Build history of the part. All positions in model axes, mm. A direction names the side the tool comes from. Give positions to 0.01 mm unless a question says otherwise; leave off trailing zeros. Loops run counter-clockwise (first coordinate to the right, second up) from the corner with the lowest first, then second, coordinate; pieces in that order, holes last.
1) Two-plate mould, pull along Z, no slides. Class faces 3 (the flat face through (-5.836, -5, -16)), 4 (the cylindrical face through (-6.44, 63.89, -17.02)), 5 (the flat face through (-29, -6, 0)), 6 (the cylindrical face through (-6.428, -82.873, -27.291)): +Z half, -Z half, draft (parallel to the pull), parting line (faces both ways), or undercut.
2) 3-axis set-ups, long thin cutter, end or side, ignore diameter. For faces 1 (the flat face through (-29, -6, -1.2)), 2 (the cylindrical face through (-51.63, 75.05, -16.89)): which of +Z, -Z, +X, -X, +Y, -Y reach the whole face in a straight line?
3) Flat gauge pins, fed straight in: P1, Ø0.6, axis at x = -6.5, y = 48.5, coming from the +Z side; P2, Ø1, axis at x = -29, z = -0.5, coming from the +Y side; P3, Ø6, axis at x = -34.5, y = -4.5, coming from the -Z side. Where does each tip first touch, or does it go through?
4) Band-saw the part on A-A on y = 20. List the corners of the cut face in (x, z), then the cut area to 3 significant figures.
5) Band-saw the part on B-B on x = -33. List the corners of the cut face in (y, z).
6) Wall check: line 1 (X direction, y = -3, z = -16.5); line 2 (Z direction, x = -39, y = -20). Give the ranges that are in metal, low to high.
```python
from build123d import *

# Parameters (mm, degrees)
SKETCH_1_W                         = 44
SKETCH_1_H                         = 100
SM_BASE_FLANGE_1_DEPTH             = 1.2
SM_EDGE_FLANGE_2_STRIP_W           = 6.2732
SM_EDGE_FLANGE_2_STRIP_H           = 1.2
SM_EDGE_FLANGE_2_STRIP_CUT_DEPTH   = 100
SM_EDGE_FLANGE_2_STRIP_2_W         = 6.2732
SM_EDGE_FLANGE_2_STRIP_2_H         = 1.2
SM_EDGE_FLANGE_2_STRIP_CUT_2_DEPTH = 100
SM_EDGE_FLANGE_2_DEPTH             = 100
SM_EDGE_FLANGE_2_BEND_DEPTH        = 100
EXTRUDE_1_DEPTH                    = 1.2
EXTRUDE_START                      = -1.2
EXTRUDE_2_DEPTH                    = 1.2
SKETCH_44_R                        = 3.5
CUT_EXTRUDE_3_DEPTH                = 94.590588423
SKETCH_45_W                        = 1.2
SKETCH_45_H                        = 29.2634
EXTRUDE_3_DEPTH                    = 30
SKETCH_48_R                        = 3.5
CUT_EXTRUDE_4_DEPTH                = 104.065268641
FILLET_1_R                         = 13


# Sheet-metal steps are written as plain solids
with BuildPart() as part:
    # Sketch 1 → 基材-凸緣1 (new body)
    with BuildSketch(Plane.XY):
        with Locations((-29.036181479, -6.57972973)):
            Rectangle(SKETCH_1_W, SKETCH_1_H)
    extrude(amount=-SM_BASE_FLANGE_1_DEPTH)

    # 邊線-凸緣2 strip (across the edge) → 邊線-凸緣2 strip cut (cut)
    with BuildSketch(Plane(origin=(-7.036181479, 43.42027027, -1.2), x_dir=(-1, 0, 0), z_dir=(0, -1, 0))):
        with Locations((-2.4, -0.6)):
            Rectangle(SM_EDGE_FLANGE_2_STRIP_W, SM_EDGE_FLANGE_2_STRIP_H)
    extrude(amount=SM_EDGE_FLANGE_2_STRIP_CUT_DEPTH, mode=Mode.SUBTRACT)

    # 邊線-凸緣2 strip 2 (across the edge) → 邊線-凸緣2 strip cut 2 (cut)
    with BuildSketch(Plane(origin=(-51.036181479, -56.57972973, -1.2), x_dir=(1, 0, 0), z_dir=(0, 1, 0))):
        with Locations((-2.4, -0.6)):
            Rectangle(SM_EDGE_FLANGE_2_STRIP_2_W, SM_EDGE_FLANGE_2_STRIP_2_H)
    extrude(amount=SM_EDGE_FLANGE_2_STRIP_CUT_2_DEPTH, mode=Mode.SUBTRACT)

    # 邊線-凸緣2 section (across the edge) → 邊線-凸緣2 (add)
    with BuildSketch(Plane(origin=(-7.036181479, 43.42027027, -1.2), x_dir=(-1, 0, 0), z_dir=(0, -1, 0))):
        with BuildLine():
            Line((-1.2, 0.7366), (-1.2, 30))
            Line((-1.2, 30), (0, 30))
            Line((0, 30), (0, 0.7366))
            ThreePointArc((0, 0.7366), (0.215745145, 0.215745145), (0.7366, 0))
            Line((0.7366, 0), (0.7366, -1.2))
            ThreePointArc((0.7366, -1.2), (-0.632782992, -0.632782992), (-1.2, 0.7366))
        make_face()
    extrude(amount=SM_EDGE_FLANGE_2_DEPTH)

    # 邊線-凸緣2 section 2 (across the edge) → 邊線-凸緣2 bend (add)
    with BuildSketch(Plane(origin=(-51.036181479, -56.57972973, -1.2), x_dir=(1, 0, 0), z_dir=(0, 1, 0))):
        with BuildLine():
            Line((-1.2, 0.7366), (-1.2, 30))
            Line((-1.2, 30), (0, 30))
            Line((0, 30), (0, 0.7366))
            ThreePointArc((0, 0.7366), (0.215745145, 0.215745145), (0.7366, 0))
            Line((0.7366, 0), (0.7366, -1.2))
            ThreePointArc((0.7366, -1.2), (-0.632782992, -0.632782992), (-1.2, 0.7366))
        make_face()
    extrude(amount=SM_EDGE_FLANGE_2_BEND_DEPTH)

    # 草圖38 → 填料-伸長1 (add)
    with BuildSketch(Plane(origin=(-5.836181479, 0, 0), x_dir=(0, 0, -1), z_dir=(1, 0, 0))):
        with BuildLine():
            Line((1.9366, 43.42027027), (31.2, 43.42027027))
            Line((31.2, 43.42027027), (31.2, 60.42027027))
            ThreePointArc((31.2, 60.42027027), (16.5683, 75.05197027), (1.9366, 60.42027027))
            Line((1.9366, 60.42027027), (1.9366, 43.42027027))
        make_face()
    extrude(amount=-EXTRUDE_1_DEPTH)

    # 草圖41 → 填料-伸長2 (add)
    with BuildSketch(Plane.ZY.offset(52.236181479).offset(EXTRUDE_START)):
        with BuildLine():
            Line((-1.9366, 43.42027027), (-31.2, 43.42027027))
            Line((-31.2, 43.42027027), (-31.2, 60.42027027))
            ThreePointArc((-31.2, 60.42027027), (-16.5683, 75.05197027), (-1.9366, 60.42027027))
            Line((-1.9366, 60.42027027), (-1.9366, 43.42027027))
        make_face()
    extrude(amount=EXTRUDE_2_DEPTH)

    # 草圖44 → 除料-伸長3 (cut, through all)
    with BuildSketch(Plane.ZY.offset(52.236181479)):
        with Locations((-16.5683, 60.42027027)):
            Circle(SKETCH_44_R)
        with BuildLine():
            ThreePointArc((-13.204663636, 69.037024323), (-16.5683, 69.67027027), (-19.931936364, 69.037024323))
            ThreePointArc((-19.931936364, 69.037024323), (-20.499840979, 67.741846981), (-19.204663636, 67.173942366))
            ThreePointArc((-19.204663636, 67.173942366), (-16.5683, 67.67027027), (-13.931936364, 67.173942366))
            ThreePointArc((-13.931936364, 67.173942366), (-12.636759021, 67.741846981), (-13.204663636, 69.037024323))
        make_face()
        with BuildLine():
            ThreePointArc((-7.951545947, 57.056633907), (-7.3183, 60.42027027), (-7.951545947, 63.783906634))
            ThreePointArc((-7.951545947, 63.783906634), (-9.246723289, 64.351811249), (-9.814627904, 63.056633907))
            ThreePointArc((-9.814627904, 63.056633907), (-9.3183, 60.42027027), (-9.814627904, 57.783906634))
            ThreePointArc((-9.814627904, 57.783906634), (-9.246723289, 56.488729292), (-7.951545947, 57.056633907))
        make_face()
        with BuildLine():
            ThreePointArc((-19.931936364, 51.803516217), (-16.5683, 51.17027027), (-13.204663636, 51.803516217))
            ThreePointArc((-13.204663636, 51.803516217), (-12.636759021, 53.098693559), (-13.931936364, 53.666598175))
            ThreePointArc((-13.931936364, 53.666598175), (-16.5683, 53.17027027), (-19.204663636, 53.666598175))
            ThreePointArc((-19.204663636, 53.666598175), (-20.499840979, 53.098693559), (-19.931936364, 51.803516217))
        make_face()
        with BuildLine():
            ThreePointArc((-25.185054053, 63.783906634), (-25.8183, 60.42027027), (-25.185054053, 57.056633907))
            ThreePointArc((-25.185054053, 57.056633907), (-23.889876711, 56.488729292), (-23.321972096, 57.783906634))
            ThreePointArc((-23.321972096, 57.783906634), (-23.8183, 60.42027027), (-23.321972096, 63.056633907))
            ThreePointArc((-23.321972096, 63.056633907), (-23.889876711, 64.351811249), (-25.185054053, 63.783906634))
        make_face()
    extrude(amount=-CUT_EXTRUDE_3_DEPTH, mode=Mode.SUBTRACT)

    # 草圖45 → 填料-伸長3 (add)
    with BuildSketch(Plane.XZ.offset(56.57972973)):
        with Locations((-51.636181479, -16.5683)):
            Rectangle(SKETCH_45_W, SKETCH_45_H)
        with Locations((-6.436181479, -16.5683)):
            Rectangle(SKETCH_45_W, SKETCH_45_H)
    extrude(amount=EXTRUDE_3_DEPTH)

    # 草圖48 → 除料-伸長4 (cut, through all)
    with BuildSketch(Plane.ZY.offset(52.236181479)):
        with Locations((-16.5683, -71.57972973)):
            Circle(SKETCH_48_R)
        with BuildLine():
            ThreePointArc((-7.951545947, -74.943366093), (-7.3183, -71.57972973), (-7.951545947, -68.216093366))
            ThreePointArc((-7.951545947, -68.216093366), (-9.246723289, -67.648188751), (-9.814627904, -68.943366093))
            ThreePointArc((-9.814627904, -68.943366093), (-9.3183, -71.57972973), (-9.814627904, -74.216093366))
            ThreePointArc((-9.814627904, -74.216093366), (-9.246723289, -75.511270708), (-7.951545947, -74.943366093))
        make_face()
        with BuildLine():
            ThreePointArc((-19.204663636, -78.333401825), (-16.5683, -78.82972973), (-13.931936364, -78.333401825))
            ThreePointArc((-13.931936364, -78.333401825), (-12.636759021, -78.901306441), (-13.204663636, -80.196483783))
            ThreePointArc((-13.204663636, -80.196483783), (-16.5683, -80.82972973), (-19.931936364, -80.196483783))
            ThreePointArc((-19.931936364, -80.196483783), (-20.499840979, -78.901306441), (-19.204663636, -78.333401825))
        make_face()
        with BuildLine():
            ThreePointArc((-23.321972096, -68.943366093), (-23.8183, -71.57972973), (-23.321972096, -74.216093366))
            ThreePointArc((-23.321972096, -74.216093366), (-23.889876711, -75.511270708), (-25.185054053, -74.943366093))
            ThreePointArc((-25.185054053, -74.943366093), (-25.8183, -71.57972973), (-25.185054053, -68.216093366))
            ThreePointArc((-25.185054053, -68.216093366), (-23.889876711, -67.648188751), (-23.321972096, -68.943366093))
        make_face()
        with BuildLine():
            ThreePointArc((-13.931936364, -64.826057634), (-16.5683, -64.32972973), (-19.204663636, -64.826057634))
            ThreePointArc((-19.204663636, -64.826057634), (-20.499840979, -64.258153019), (-19.931936364, -62.962975677))
            ThreePointArc((-19.931936364, -62.962975677), (-16.5683, -62.32972973), (-13.204663636, -62.962975677))
            ThreePointArc((-13.204663636, -62.962975677), (-12.636759021, -64.258153019), (-13.931936364, -64.826057634))
        make_face()
    extrude(amount=-CUT_EXTRUDE_4_DEPTH, mode=Mode.SUBTRACT)

    # 圓角1
    fillet_1_edges = [part.edges().sort_by_distance(p)[0] for p in [
        (-51.636181479, -86.57972973, -31.2),
        (-51.636181479, -86.57972973, -1.9366),
        (-6.436181479, -86.57972973, -31.2),
        (-6.436181479, -86.57972973, -1.9366),
    ]]
    fillet(fillet_1_edges, radius=FILLET_1_R)


solid = part.part
```
Findings below:
1. face 3: draft
1. face 4: undercut
1. face 5: +Z half
1. face 6: -Z half
2. face 1: -Z, +Y, -Y
2. face 2: +X, -X, +Y
3. P1: stops at z = -1.94
3. P2: stops at y = 43.42
3. P3: stops at z = -1.2
4. outline: (-52.24, -31.2) - (-51.04, -31.2) - (-51.04, -1.94) arc R0.74 cw to (-50.3, -1.2) - (-7.77, -1.2) arc R0.74 cw to (-7.04, -1.94) - (-7.04, -31.2) - (-5.84, -31.2) - (-5.84, -1.94) arc R1.94 ccw to (-7.77, 0) - (-50.3, 0) arc R1.94 ccw to (-52.24, -1.94) - close
4. area: 126 mm2
5. outline: (-56.58, -1.2) - (43.42, -1.2) - (43.42, 0) - (-56.58, 0) - close
6. line 1: x = -52.24 to -51.04, -7.04 to -5.84
6. line 2: z = -1.2 to 0
